Geometry: final body of the model. Coordinates: model frame, mm. A direction names the side the tool comes from. Give positions to 0.01 mm unless a question says otherwise; leave off trailing zeros. Write each loop counter-clockwise with the first axis right and the second up, starting at its lowest first coordinate (ties: lowest second). Pieces come first, ordered by that corner, then holes. Notation, with made-up numbers: (30.25, 33.25) - (82.25, 33.25) arc R9 cw to (82.25, 38.25) - close; hole circle Ø5 at (37.5, -12.75). An arc over 180 degrees is marked (long way). Return JSON: item names as keys, results as strings.
from build123d import *

# Parameters (mm, degrees)
F2_W     = 56
F2_H     = 56
F2_W_2   = 50
F2_H_2   = 50
F3_DEPTH = 100
F4_DEPTH = 3
F5_W     = 20
F5_H     = 20
F6_DEPTH = 3
F7_W     = 3
F7_H     = 25
F8_DEPTH = 3


with BuildPart() as f3:
    # F2 (on Top) → F3 (new body)
    with BuildSketch(Plane.XY):
        with Locations((28, 28)):
            Rectangle(F2_W, F2_H)
        with Locations((28, 28)):
            Rectangle(F2_W_2, F2_H_2, mode=Mode.SUBTRACT)
    extrude(amount=F3_DEPTH)

    # F2 (on Top) → F4 (join)
    with BuildSketch(Plane.XY):
        with Locations((28, 28)):
            Rectangle(F2_W, F2_H)
        with Locations((28, 28)):
            Rectangle(F2_W_2, F2_H_2, mode=Mode.SUBTRACT)
        with Locations((28, 28)):
            Rectangle(F2_W_2, F2_H_2)
    extrude(amount=-F4_DEPTH)

    # F5 (on face) → F6 (cut, through all)
    with BuildSketch(Plane.XY):
        with Locations((13, 13)):
            Rectangle(F5_W, F5_H)
    extrude(amount=-F6_DEPTH, mode=Mode.SUBTRACT)

    # F7 (on face) → F8 (cut, through all)
    with BuildSketch(Plane(origin=(0, 56, 0), x_dir=(-1, 0, 0), z_dir=(0, 1, 0))):
        with Locations((-47.5, 48.5)):
            Rectangle(F7_W, F7_H)
        with Locations((-8.5, 48.5)):
            Rectangle(F7_W, F7_H)
    extrude(amount=-F8_DEPTH, mode=Mode.SUBTRACT)


solid = f3.part
Q1. Material intervals for probe 1 along X at (y, z) = (9.5, 19); probe 2 along Z at (x, y) = (16, 35.5), sorted ascending. Write a range as [from, to].
Answer key:
{"probe 1": "x = [0, 3], [53, 56]", "probe 2": "z = [-3, 0]"}
Q2. Set-up query: faces 5 (the flat face through (28, 28, -3)), 6 (the flat face through (28, 3, 49)), 7 (the flat face through (9, 55, 61)), 8 (the flat face through (13, 23, -1)). Return all of +Z, -Z, +X, -X, +Y, -Y with unobstructed straight access to the full face (end or side cutting, diameter ignored); none if empty.
Answer key:
{"face 5": "-Z, +X, -X, +Y, -Y", "face 6": "+Z", "face 7": "+Y", "face 8": "+Z, -Z"}
Q3. Section query B-B, the plane z = 49.5. Return the cut outline in (x, y).
Answer key:
{"outline": "(0, 0) - (56, 0) - (56, 56) - (49, 56) - (49, 53) - (53, 53) - (53, 3) - (3, 3) - (3, 53) - (7, 53) - (7, 56) - (0, 56) - close; (10, 53) - (46, 53) - (46, 56) - (10, 56) - close"}
Q4. Mould query, pull axis X, two halves, no side actions, for faces 1 (the flat face through (48, 55, 61)), 2 (the flat face through (56, 28, 49)), 3 (the flat face through (28, 0, 49)), 4 (the flat face through (46, 55, 48)). Classes: pulls with the +X half, pulls with the -X half, needs draft (parallel to the pull), parting line crosses it, or undercut.
Answer key:
{"face 1": "undercut", "face 2": "pulls with the +X half", "face 3": "needs draft", "face 4": "undercut"}
Q5. Pin query (flat end, axial travel): P1, Ø4, axis at x = 49.5, y = 45.5, coming from the +Z side. Return the tip coordinate at first contact, or that it passes through.
Answer key:
{"P1": "stops at z = 0"}
Q6. Section query A-A, the plane y = 18.5. Return the cut outline in (x, z), plus the area to 3 significant figures.
Answer key:
{"outline": "(0, -3) - (3, -3) - (3, 100) - (0, 100) - close; (23, -3) - (56, -3) - (56, 100) - (53, 100) - (53, 0) - (23, 0) - close", "area": "708 mm^2"}
Q7. Section query D-D, the plane z = 23.5. Return the cut outline in (x, y).
Answer key:
{"outline": "(0, 0) - (56, 0) - (56, 56) - (0, 56) - close; hole (3, 3) - (53, 3) - (53, 53) - (3, 53) - close"}
